Design review of the part built by this model. Coordinates are the model's own, in mm. A direction names the side the tool comes from. Coordinates: 2 decimals unless noted, no trailing zeros. Write each loop counter-clockwise with the first axis right and the second up, starting at its lowest first coordinate (ties: lowest second). Pieces come first, ordered by that corner, then holes.
Q1. Take a section at B-B, the plane x = 108. Write out the cut boundary in (y, z), plus the area to 3 significant figures.
Q2. Take a section at D-D, the plane z = -9. Write out the cut boundary in (x, y).
Q3. The part is to be moulded in two halves that separate along X. For faces 5 (the flat face through (72, -4, 2.54)), 6 (the flat face through (-16.75, -49, -11)), 7 (the flat face through (72, -2, 0)), say which applies: released by +X, released by -X, zero draft, split by the parting line, or undercut.
Q4. For L1, parallel to X at y = -30, z = 60; L2, parallel to X at y = -66.5, z = -11.5; L3, parallel to Y at x = 39.5, z = 4, list the stretches that pass through material, from the lowest coordinate up.
Q5. For faces 1 (the flat face through (71, -2.54, -11)), 2 (the flat face through (162.208, -48, -11)), 3 (the flat face through (162.208, -48, 43)), 4 (the flat face through (72, -5.08, -10)), list the 3-axis set-ups (+Z, -Z, +X, -X, +Y, -Y) from which the entire face can be reached by the end or side of a thin tool; tool diameter is ignored.
Q6. Take a section at A-A, the plane z = 8.5. Write out the cut boundary in (x, y).
Q7. Take a section at C-C, the plane y = -76.5. Write out the cut boundary in (x, z).
Q8. For pin 1 Ø12.5 at (y, z) = (-39, -10) entering from -X; pin 2 Ø4 at (x, y) = (77, -63.5) entering from -Z; pin 3 Ø20.5 at (x, z) = (61, -15) entering from -Y, all flat-tipped, find the tip position at first contact; note any pin that passes through.
from build123d import *

# Parameters (mm, degrees)
F0_W        = 184.0382497758
F0_H        = 87.4423235655
F1_DEPTH    = 94.488
F2_T        = -2.54
F3_DEPTH    = 25.4
F4_T        = 2.54
F4_T3_DEPTH = 97.028
F4_T5_DEPTH = 184.0382497758
F4_T7_DEPTH = 87.4423235655


# Not quite as in the source:
# - a shell that OpenCascade refuses in one call is made with other operations: the cavity is built on its own and cut out


with BuildPart() as f1:
    # F0 (on Front) → F1 (new body)
    with BuildSketch(Plane.XZ):
        with Locations((72.7289924398, 43.7211617827)):
            Rectangle(F0_W, F0_H)
    extrude(amount=F1_DEPTH)

    # F2
    f2_openings = [f1.faces().sort_by_distance(p)[0] for p in [
        (72.728992, -94.488, 43.721162),
    ]]
    offset(amount=F2_T, openings=f2_openings)

    # F3 (add): a face of the model
    f3_faces = [f1.faces().sort_by_distance(p)[0] for p in [
        (72.7289924398, -48.514, 2.54),
    ]]
    extrude(f3_faces, amount=-F3_DEPTH)

    # F4: shell of thickness 2.54, made by hand


with BuildPart() as f4_core1:
    # F4_t2: copy of F1
    add(f1.part)

    # the walls: a layer under each face that stays
    f4_faces = [f4_core1.faces().sort_by_distance(p)[0] for p in [
        (-19.2901324481, -47.244, 43.7211617827),
        (72.7289924398, -47.244, 87.4423235655),
        (104.36056662, -2.333037037, 0),
        (72.7289924398, 0, 43.7211617827),
        (164.7481173277, -47.244, 43.7211617827),
        (162.2081173277, -48.514, -11.43),
        (72.7289924398, -2.54, -11.43),
        (-16.7501324481, -48.514, -11.43),
        (162.2081173277, -48.514, 43.7211617827),
        (72.7289924398, -48.514, 84.9023235655),
        (-16.7501324481, -48.514, 43.7211617827),
        (72.7289924398, -2.54, 43.7211617827),
    ]]
    thicken(f4_faces, amount=-F4_T, mode=Mode.SUBTRACT)

    # F4_s4 → F4_t3 (cut)
    with BuildSketch(Plane.XZ):
        Polygon((162.2335173277, -0.0254), (162.2081173277, 2.54), (159.6681173277, 2.54), (159.6681173277, 0), align=None)
        Polygon((-16.7755324481, -0.0254), (-16.7501324481, 2.54), (-14.2101324481, 2.54), (-14.2101324481, 0), align=None)
        Polygon((162.1827173277, 84.8769235655), (164.7481173277, 84.9023235655), (164.7481173277, 87.4423235655), (162.2081173277, 87.4423235655), align=None)
        Polygon((-16.7247324481, 84.8769235655), (-16.7501324481, 87.4423235655), (-19.2901324481, 87.4423235655), (-19.2901324481, 84.9023235655), align=None)
    extrude(amount=F4_T3_DEPTH, mode=Mode.SUBTRACT)

    # F4_s6 → F4_t5 (cut)
    with BuildSketch(Plane.YZ.offset(-19.2901324481)):
        Polygon((-2.5146, -0.0254), (-2.54, 2.54), (-5.08, 2.54), (-5.08, 0), align=None)
        Polygon((-2.5654, 84.8769235655), (-2.54, 87.4423235655), (0, 87.4423235655), (0, 84.9023235655), align=None)
    extrude(amount=F4_T5_DEPTH, mode=Mode.SUBTRACT)

    # F4_s8 → F4_t7 (cut)
    with BuildSketch(Plane.XY):
        Polygon((162.1827173277, -2.5654), (164.7481173277, -2.54), (164.7481173277, 0), (162.2081173277, 0), align=None)
        Polygon((-16.7247324481, -2.5654), (-19.2901324481, -2.54), (-19.2901324481, 0), (-16.7501324481, 0), align=None)
    extrude(amount=F4_T7_DEPTH, mode=Mode.SUBTRACT)


with BuildPart() as f1_1:
    add(f1.part)

    # what is left inside the walls is the cavity
    f4_cavity = [f4_core1.part.solids().sort_by_distance(p)[0] for p in [
        (72.728992, -64.685333, 2.5146),
    ]]
    add(f4_cavity, mode=Mode.SUBTRACT)


solid = f1_1.part
Responses:
1. outline: (-94.49, 84.9) - (-2.54, 84.9) - (-2.54, 2.54) - (-5.08, 2.54) - (-5.08, -22.86) - (-2.54, -22.86) - (-2.54, 0) - (0, 0) - (0, 87.44) - (-94.49, 87.44) - close
1. area: 520 mm2
2. outline: (-16.75, -94.49) - (-14.21, -94.49) - (-14.21, -5.08) - (159.67, -5.08) - (159.67, -94.49) - (162.21, -94.49) - (162.21, -2.54) - (-16.75, -2.54) - close
3. face 5: undercut
3. face 6: released by -X
3. face 7: zero draft
4. L1: x = -19.29 to -16.75, 162.21 to 164.75
4. L2: x = -16.75 to -14.21, 159.67 to 162.21
4. L3: y = -2.54 to 0
5. face 1: -Z, +X, -X, +Y
5. face 2: -Z, +X, +Y, -Y
5. face 3: -Y
5. face 4: -Z, -Y
6. outline: (-19.29, -94.49) - (-16.75, -94.49) - (-16.75, -2.54) - (162.21, -2.54) - (162.21, -94.49) - (164.75, -94.49) - (164.75, 0) - (-19.29, 0) - close
7. outline: (-19.29, 0) - (-16.75, 0) - (-16.75, -22.86) - (-14.21, -22.86) - (-14.21, 2.54) - (-16.75, 2.54) - (-16.75, 84.9) - (162.21, 84.9) - (162.21, 2.54) - (159.67, 2.54) - (159.67, -22.86) - (162.21, -22.86) - (162.21, 0) - (164.75, 0) - (164.75, 87.44) - (-19.29, 87.44) - close
8. pin 1: stops at x = -16.75
8. pin 2: stops at z = 84.9
8. pin 3: stops at y = -5.08
